Verification items for the finished model (mm, model axes). Face numbers are marked on the shaded views. A direction names the side the tool comes from. Give positions to 0.01 mm unless a question says otherwise; leave off trailing zeros. Loops run counter-clockwise (first coordinate to the right, second up) from the corner with the lowest first, then second, coordinate; pieces in that order, holes last. Notation, with made-up numbers: M 6,31 L 62,31 A18 cw 62,42 Z; hole C -27,13 d1. An arc over 180 degrees is marked long. Use CSV: the item, a comma, the result in double quotes.
from build123d import *

# Parameters (mm, degrees)
SKETCH_1_W            = 30
SKETCH_1_H            = 30
SKETCH_1_R            = 9.807439468
EXTRUDE_1_DEPTH       = 60
SKETCH_2_W            = 30
SKETCH_2_H            = 30
SKETCH_2_R            = 10.25
EXTRUDE_2_DEPTH       = 50
SKETCH_6_R            = 10.25
CUT_EXTRUDE_1_DEPTH   = 60
SKETCH_7_W            = 30
SKETCH_7_H            = 30
SKETCH_7_R            = 10.25
REVOLVE_1_ANGLE       = 90
FILLET_2_R            = 15
SKETCH_9_W            = 65.452723958
SKETCH_9_H            = 141.93468868
CUT_EXTRUDE_3_DEPTH   = 30
SKETCH_19_W           = 90
SKETCH_19_H           = 60
EXTRUDE_9_DEPTH       = 4.5
SKETCH_20_W           = 5
SKETCH_20_H           = 60
EXTRUDE_10_DEPTH      = 15
EXTRUDE_11_DEPTH      = 25
EXTRUDE_11_DEPTH_BACK = 50
SKETCH_22_R           = 15
SKETCH_22_R_2         = 10.25
SKETCH_26_W           = 90
SKETCH_26_H           = 15
CUT_EXTRUDE_4_DEPTH   = 20
FILLET_4_R            = 3


with BuildPart() as part:
    # Sketch 1 → Extrude 1 (new body)
    with BuildSketch(Plane.XY):
        Rectangle(SKETCH_1_W, SKETCH_1_H)
        Circle(SKETCH_1_R, mode=Mode.SUBTRACT)
    extrude(amount=EXTRUDE_1_DEPTH)

    # Sketch 6 → Cut-Extrude 1 (cut)
    with BuildSketch(Plane.XY.offset(60)):
        Circle(SKETCH_6_R)
    extrude(amount=-CUT_EXTRUDE_1_DEPTH, mode=Mode.SUBTRACT)



with BuildPart() as body_2:
    # Sketch 2 → Extrude 2 (new body)
    with BuildSketch(Plane.XZ.offset(15)):
        with Locations((0, 75)):
            Rectangle(SKETCH_2_W, SKETCH_2_H)
        with Locations((0, 75)):
            Circle(SKETCH_2_R, mode=Mode.SUBTRACT)
    extrude(amount=EXTRUDE_2_DEPTH)


with BuildPart() as part_1:
    add(part.part)

    add(body_2.part)  # Revolve 1 merges body 2
    # Sketch 7 → Revolve 1 (revolve)
    with BuildSketch(Plane(origin=(0, -15, 0), x_dir=(1, 0, 0), z_dir=(0, 1, 0))):
        with Locations((0, -75)):
            Rectangle(SKETCH_7_W, SKETCH_7_H)
        with Locations(Location((0, -75, 0), (0, 0, 270))):
            Circle(SKETCH_7_R, mode=Mode.SUBTRACT)
    revolve(axis=Axis((15, -15, 60), (-1, 0, 0)), revolution_arc=REVOLVE_1_ANGLE)

    # Fillet 2
    # the kernel refuses this fillet: 15 mm, written as the material it adds along each edge
    with BuildSketch(Plane(origin=(15, -15, 60), x_dir=(0, 0, -1), z_dir=(-1, 0, 0))) as fillet_2_piece_1:
        with BuildLine():
            CenterArc((FILLET_2_R, FILLET_2_R), FILLET_2_R, 180, 90)
            Line((0, FILLET_2_R), (0, 0))
            Line((0, 0), (FILLET_2_R, 0))
        make_face()
    extrude(amount=30)
    # the kernel refuses this fillet: 15 mm, written as the material it takes off along each edge
    with BuildSketch(Plane(origin=(15, -15, 60), x_dir=(0, 0, 1), z_dir=(0, -1, 0))) as fillet_2_2_piece_1:
        with BuildLine():
            CenterArc((30 - FILLET_2_R, FILLET_2_R), FILLET_2_R, 270, 90)
            Line((30, FILLET_2_R), (30, 0))
            Line((30, 0), (30 - FILLET_2_R, 0))
        make_face()
    revolve(axis=Axis((15, -15, 60), (-1, 0, 0)), revolution_arc=90, mode=Mode.SUBTRACT)
    with BuildSketch(Plane(origin=(-15, -15, 60), x_dir=(0, 0, 1), z_dir=(0, -1, 0))) as fillet_2_2_piece_2:
        with BuildLine():
            CenterArc((30 - FILLET_2_R, -FILLET_2_R), FILLET_2_R, 0, 90)
            Line((30, -FILLET_2_R), (30, 0))
            Line((30, 0), (30 - FILLET_2_R, 0))
        make_face()
    revolve(axis=Axis((-15, -15, 60), (-1, 0, 0)), revolution_arc=90, mode=Mode.SUBTRACT)
    with BuildSketch(Plane(origin=(-15, 15, -37.5), x_dir=(0, -1, 0), z_dir=(0, 0, 1))) as fillet_2_2_piece_3:
        with BuildLine():
            CenterArc((FILLET_2_R, FILLET_2_R), FILLET_2_R, 180, 90)
            Line((0, FILLET_2_R), (0, 0))
            Line((0, 0), (FILLET_2_R, 0))
        make_face()
    extrude(amount=97.5, mode=Mode.SUBTRACT)
    with BuildSketch(Plane(origin=(15, 15, -37.5), x_dir=(0, -1, 0), z_dir=(0, 0, 1))) as fillet_2_2_piece_4:
        with BuildLine():
            CenterArc((FILLET_2_R, -FILLET_2_R), FILLET_2_R, 90, 90)
            Line((0, -FILLET_2_R), (0, 0))
            Line((0, 0), (FILLET_2_R, 0))
        make_face()
    extrude(amount=97.5, mode=Mode.SUBTRACT)
    with BuildSketch(Plane(origin=(-15, -15, 90), x_dir=(0, 0, -1), z_dir=(0, -1, 0))) as fillet_2_2_piece_5:
        with BuildLine():
            CenterArc((FILLET_2_R, FILLET_2_R), FILLET_2_R, 180, 90)
            Line((0, FILLET_2_R), (0, 0))
            Line((0, 0), (FILLET_2_R, 0))
        make_face()
    extrude(amount=87.5, mode=Mode.SUBTRACT)
    with BuildSketch(Plane(origin=(15, -15, 90), x_dir=(0, 0, -1), z_dir=(0, -1, 0))) as fillet_2_2_piece_6:
        with BuildLine():
            CenterArc((FILLET_2_R, -FILLET_2_R), FILLET_2_R, 90, 90)
            Line((0, -FILLET_2_R), (0, 0))
            Line((0, 0), (FILLET_2_R, 0))
        make_face()
    extrude(amount=87.5, mode=Mode.SUBTRACT)
    # the kernel refuses this fillet: 15 mm, written as the material it takes off along each edge
    with BuildSketch(Plane(origin=(-15, -15, 45), x_dir=(1, 0, 0), z_dir=(0, 0, -1)), Plane(origin=(15, -15, -37.5), x_dir=(-1, 0, 0), z_dir=(0, 0, 1))) as fillet_2_3_piece_1:
        with BuildLine():
            CenterArc((FILLET_2_R, -FILLET_2_R), FILLET_2_R, 90, 90)
            Line((0, -FILLET_2_R), (0, 0))
            Line((0, 0), (FILLET_2_R, 0))
        make_face()
    extrude(amount=82.5, mode=Mode.SUBTRACT)
    with BuildSketch(Plane(origin=(15, -30, 60), x_dir=(0, 0, 1), z_dir=(0, -1, 0))) as fillet_2_3_piece_2:
        with BuildLine():
            CenterArc((FILLET_2_R, FILLET_2_R), FILLET_2_R, 180, 90)
            Line((0, FILLET_2_R), (0, 0))
            Line((0, 0), (FILLET_2_R, 0))
        make_face()
    extrude(amount=72.5, mode=Mode.SUBTRACT)
    with BuildSketch(Plane(origin=(-15, -30, 60), x_dir=(0, 0, 1), z_dir=(0, -1, 0))) as fillet_2_3_piece_3:
        with BuildLine():
            CenterArc((FILLET_2_R, -FILLET_2_R), FILLET_2_R, 90, 90)
            Line((0, -FILLET_2_R), (0, 0))
            Line((0, 0), (FILLET_2_R, 0))
        make_face()
    extrude(amount=72.5, mode=Mode.SUBTRACT)
    with BuildSketch(Plane(origin=(-15, -30, 45), x_dir=(0, 1, 0), z_dir=(0, 0, -1))) as fillet_2_3_piece_4:
        with BuildLine():
            CenterArc((15 + FILLET_2_R, FILLET_2_R), FILLET_2_R, 180, 90)
            Line((15, FILLET_2_R), (15, 0))
            Line((15, 0), (15 + FILLET_2_R, 0))
        make_face()
    revolve(axis=Axis((-15, -30, 45), (1, 0, 0)), revolution_arc=90, mode=Mode.SUBTRACT)
    with BuildSketch(Plane(origin=(15, -30, 45), x_dir=(0, 1, 0), z_dir=(0, 0, -1))) as fillet_2_3_piece_5:
        with BuildLine():
            CenterArc((15 + FILLET_2_R, -FILLET_2_R), FILLET_2_R, 90, 90)
            Line((15 + FILLET_2_R, 0), (15, 0))
            Line((15, 0), (15, -FILLET_2_R))
        make_face()
    revolve(axis=Axis((15, -30, 45), (1, 0, 0)), revolution_arc=90, mode=Mode.SUBTRACT)

    # Sketch 9 → Cut-Extrude 3 (cut)
    with BuildSketch(Plane(origin=(15, 0, 0), x_dir=(0, 0, -1), z_dir=(1, 0, 0))):
        with Locations((-60, 0)):
            Rectangle(SKETCH_9_W, SKETCH_9_H)
    extrude(amount=-CUT_EXTRUDE_3_DEPTH, mode=Mode.SUBTRACT)

    # Sketch 19 → Extrude 9 (add)
    with BuildSketch(Plane(origin=(-15, -15, 60), x_dir=(0, 0, -1), z_dir=(1, 0, 0))):
        with Locations((46.36318099, 15)):
            Rectangle(SKETCH_19_W, SKETCH_19_H)
    extrude(amount=EXTRUDE_9_DEPTH)

    # Sketch 20 → Extrude 10 (add)
    with BuildSketch(Plane.ZY.offset(15)):
        with Locations((56.13681901, 0)):
            Rectangle(SKETCH_20_W, SKETCH_20_H)
        with Locations((-28.86318099, 0)):
            Rectangle(SKETCH_20_W, SKETCH_20_H)
    extrude(amount=EXTRUDE_10_DEPTH)

    # Sketch 22 → Extrude 11 (add, two sides: drawn at the far end of the back side and taken through both)
    with BuildSketch(Plane.XY.offset(27.273638021).offset(-EXTRUDE_11_DEPTH_BACK)):
        Circle(SKETCH_22_R)
        Circle(SKETCH_22_R_2, mode=Mode.SUBTRACT)
    extrude(amount=EXTRUDE_11_DEPTH + EXTRUDE_11_DEPTH_BACK)

    # Sketch 26 → Cut-Extrude 4 (cut)
    with BuildSketch(Plane(origin=(-10.5, 0, 0), x_dir=(0, 0, -1), z_dir=(1, 0, 0))):
        with Locations((-13.63681901, -22.5)):
            Rectangle(SKETCH_26_W, SKETCH_26_H)
        with Locations((-13.63681901, 22.5)):
            Rectangle(SKETCH_26_W, SKETCH_26_H)
    extrude(amount=-CUT_EXTRUDE_4_DEPTH, mode=Mode.SUBTRACT)

    # Fillet 4
    # the kernel refuses this fillet: 3 mm, written as the material it adds along each edge
    with BuildSketch(Plane(origin=(-10.5, -10.712142643, 27.273638021), x_dir=(0.8191977687507059, -0.573511129511769, 0), z_dir=(0, 0, -1))) as fillet_4_piece_1:
        with BuildLine():
            CenterArc((5.4076958, 2.959446042), FILLET_4_R, 169.374679788, 91.193748437)
            Line((2.459133916, 3.51260318), (2.400162678, 3.523666322))
            ThreePointArc((2.400162678, 3.523666322), (1.180415092, 1.790712258), (-0.049151866, 0.034410668))
            Line((-0.049151866, 0.034410668), (0.009832174, -0.059188921))
            ThreePointArc((0.009832174, -0.059188921), (2.458043545, 0.142769789), (4.906254916, -0.059188921))
            Line((4.906254916, -0.059188921), (4.916087091, 0))
        make_face()
    extrude(amount=27.273638021)
    with BuildSketch(Plane(origin=(-10.5, 10.712142643, 27.273638021), x_dir=(0.8191977687507056, 0.5735111295117695, 0), z_dir=(0, 0, -1))) as fillet_4_piece_2:
        with BuildLine():
            CenterArc((5.4076958, -2.959446042), FILLET_4_R, 99.431571775, 91.193748437)
            Line((2.459133916, -3.51260318), (2.400162678, -3.523666322))
            ThreePointArc((2.400162678, -3.523666322), (1.180415092, -1.790712258), (-0.049151866, -0.034410668))
            Line((-0.049151866, -0.034410668), (0.009832174, 0.059188921))
            ThreePointArc((0.009832174, 0.059188921), (2.458043545, -0.142769789), (4.906254916, 0.059188921))
            Line((4.906254916, 0.059188921), (4.916087091, 0))
        make_face()
    extrude(amount=27.273638021)
    with BuildSketch(Plane(origin=(-10.5, 10.712142643, 52.273638021), x_dir=(0, 1, 0), z_dir=(0, 0, -1))) as fillet_4_piece_3:
        with BuildLine():
            CenterArc((5.525745321, 2.732697091), FILLET_4_R, 154.43613955, 91.193748437)
            Line((2.81943066, 4.027247576), (2.765304367, 4.053138585))
            ThreePointArc((2.765304367, 4.053138585), (1.526672022, 1.931743725), (-0.042848571, 0.042))
            Line((-0.042848571, 0.042), (0, -0.06))
            ThreePointArc((0, -0.06), (2.143928679, -0.06), (4.263099598, -0.054653942))
            Line((4.263099598, -0.054653942), (4.287857357, 0))
        make_face()
    extrude(amount=25)
    with BuildSketch(Plane(origin=(-10.5, 10.712142643, -22.726361979), x_dir=(0, 1, 0), z_dir=(0, 0, 1))) as fillet_4_piece_4:
        with BuildLine():
            CenterArc((5.525745321, -2.732697091), FILLET_4_R, 114.370112013, 91.193748437)
            Line((2.81943066, -4.027247576), (2.765304367, -4.053138585))
            ThreePointArc((2.765304367, -4.053138585), (1.526672022, -1.931743725), (-0.042848571, -0.042))
            Line((-0.042848571, -0.042), (0, 0.06))
            ThreePointArc((0, 0.06), (2.143928679, 0.06), (4.263099598, 0.054653942))
            Line((4.263099598, 0.054653942), (4.287857357, 0))
        make_face()
    extrude(amount=22.726361979)
    with BuildSketch(Plane(origin=(-10.5, -10.712142643, 52.273638021), x_dir=(0.8191977687507062, -0.5735111295117684, 0), z_dir=(0, 0, -1))) as fillet_4_piece_5:
        with BuildLine():
            CenterArc((5.4076958, 2.959446042), FILLET_4_R, 169.374679788, 91.193748437)
            Line((2.459133916, 3.51260318), (2.400162678, 3.523666322))
            ThreePointArc((2.400162678, 3.523666322), (1.180415092, 1.790712258), (-0.049151866, 0.034410668))
            Line((-0.049151866, 0.034410668), (0.009832174, -0.059188921))
            ThreePointArc((0.009832174, -0.059188921), (2.458043545, 0.142769789), (4.906254916, -0.059188921))
            Line((4.906254916, -0.059188921), (4.916087091, 0))
        make_face()
    extrude(amount=25)
    with BuildSketch(Plane(origin=(-10.5, -10.712142643, -22.726361979), x_dir=(0.8191977687507059, -0.5735111295117687, 0), z_dir=(0, 0, 1))) as fillet_4_piece_6:
        with BuildLine():
            CenterArc((5.4076958, -2.959446042), FILLET_4_R, 99.431571775, 91.193748437)
            Line((2.459133916, -3.51260318), (2.400162678, -3.523666322))
            ThreePointArc((2.400162678, -3.523666322), (1.180415092, -1.790712258), (-0.049151866, -0.034410668))
            Line((-0.049151866, -0.034410668), (0.009832174, 0.059188921))
            ThreePointArc((0.009832174, 0.059188921), (2.458043545, -0.142769789), (4.906254916, 0.059188921))
            Line((4.906254916, 0.059188921), (4.916087091, 0))
        make_face()
    extrude(amount=22.726361979)


solid = part_1.part
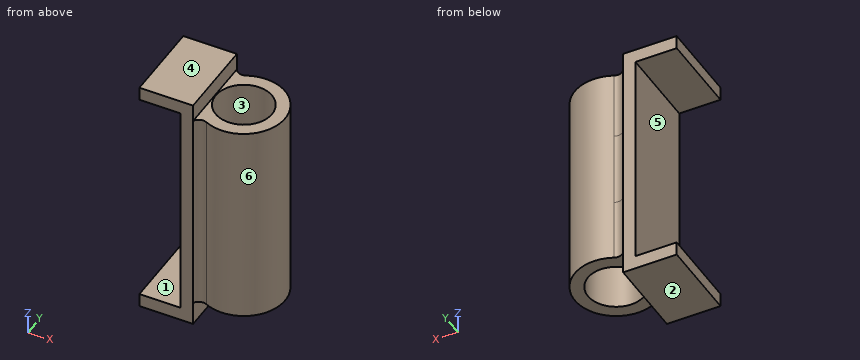
(1) Mould release check, pull along X, two halves, no side actions. Record for the marked faces 3, 4, 5 and 6: released by +X, released by -X, zero draft, split by the parting line, or undercut.
Calculated:
face 3,"undercut"
face 4,"zero draft"
face 5,"released by -X"
face 6,"undercut"
(2) Scan lines: L1, parallel to Y at x = 0, z = 32; L2, parallel to Z at x = -22.5, y = 4.5; L3, parallel to X at y = 2, z = 20. Record each from-to range of solid material in increasing order. Write a range as from..to.
Calculated:
L1,"y = -15..-10.25, 10.25..15"
L2,"z = -31.36..-26.36, 53.64..58.64"
L3,"x = -15..-10.05, 10.05..14.87"
(3) Section check D-D on x = 9. Record the cut outline in (y, z), plus the area to 3 significant figures.
Calculated:
outline,"M -12,-22.73 L -4.91,-22.73 L -4.91,52.27 L -12,52.27 Z; M 4.91,-22.73 L 12,-22.73 L 12,52.27 L 4.91,52.27 Z"
area,"1,060 mm²"
(4) Tool access check on the marked faces 1 and 2. Record the directions out of +Z, -Z, +X, -X, +Y, -Y that give a thin tool (end or side, any length) a straight path to the whole face; none if there is none.
Calculated:
face 1,"-X, +Y, -Y"
face 2,"-Z, +X, -X, +Y, -Y"
(5) Section check B-B on y = 0. Record the cut outline in (x, z), plus the area to 3 significant figures.
Calculated:
outline,"M -30,-31.36 L -10.5,-31.36 L -10.5,-22.73 L -10.25,-22.73 L -10.25,52.27 L -10.5,52.27 L -10.5,58.64 L -30,58.64 L -30,53.64 L -15,53.64 L -15,-26.36 L -30,-26.36 Z; M 10.25,-22.73 L 15,-22.73 L 15,52.27 L 10.25,52.27 Z"
area,"930 mm²"
(6) Section check C-C on z = 28.5. Record the cut outline in (x, y).
Calculated:
outline,"M -15,-15 L -10.5,-15 A3 cw -6.47,-13.53 A15 ccw long -6.47,13.53 A3 cw -10.5,15 L -15,15 Z; hole C 0,0 d20.5"
(7) Section check A-A on x = 0. Record the cut outline in (y, z).
Calculated:
outline,"M -15,-22.73 L -10.25,-22.73 L -10.25,52.27 L -15,52.27 Z; M 10.25,-22.73 L 15,-22.73 L 15,52.27 L 10.25,52.27 Z"
(8) Depth check by flat-ended pin: pin 1 Ø6 at (x, y) = (-7, -10.5) entering from -Z; pin 2 Ø13 at (x, y) = (8.5, -6) entering from +Z; pin 3 Ø15 at (y, z) = (-0.5, 32.5) entering from -X. Enter the tip coordinate at first touch or a pass-through.
Calculated:
pin 1,"stops at z = -22.73"
pin 2,"stops at z = 52.27"
pin 3,"stops at x = -15"
